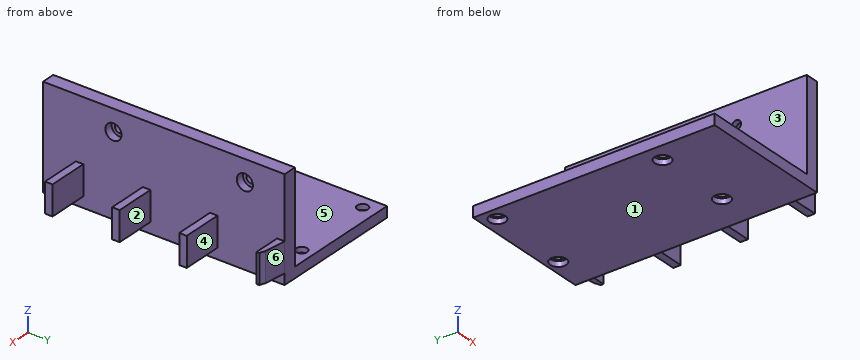
```python
from build123d import *

# Parameters (mm, degrees)
EXTRUDE_1_DEPTH     = 38
EXTRUDE_1_2_DEPTH   = 38
EXTRUDE_7_DEPTH     = 38
SKETCH_13_W         = 45
SKETCH_13_H         = 4
EXTRUDE_9_DEPTH     = 90
SKETCH_1_4_W        = 5
SKETCH_1_4_H        = 2.2
EXTRUDE_10_DEPTH    = 38
SKETCH_11_R         = 1.75
CUT_EXTRUDE_2_DEPTH = 38
CUT_EXTRUDE_START   = -2
SKETCH_11_3_R       = 3
SKETCH_11_3_R_2     = 1.75
CUT_EXTRUDE_3_DEPTH = 38
SKETCH_15_R         = 2
CUT_EXTRUDE_4_DEPTH = 38
SKETCH_15_3_R       = 3
SKETCH_15_3_R_2     = 2
CUT_EXTRUDE_5_DEPTH = 38
SKETCH_17_W         = 15
SKETCH_17_H         = 2.8
EXTRUDE_12_DEPTH    = 23
SKETCH_18_W         = 2
SKETCH_18_H         = 1
CUT_EXTRUDE_6_DEPTH = 40
SKETCH_17_2_W       = 15
SKETCH_17_2_H       = 2.8
SKETCH_17_2_W_2     = 10
SKETCH_17_2_H_2     = 3.8
CUT_EXTRUDE_7_DEPTH = 23
SKETCH_20_W         = 15
SKETCH_20_H         = 4
CUT_EXTRUDE_8_DEPTH = 89
SKETCH_17_4_W       = 5
SKETCH_17_4_H       = 10
EXTRUDE_13_DEPTH    = 38


with BuildPart() as part:
    # Sketch 1 → Extrude 1 (new body)
    with BuildSketch(Plane.XY):
        Polygon((15, -3.8), (15, -1.8), (13, -1), (13, -3.8), align=None)
    extrude(amount=EXTRUDE_1_DEPTH)



with BuildPart() as body_2:
    # Sketch 1 → Extrude 1 2 (new body)
    with BuildSketch(Plane.XY):
        Polygon((5, -75), (5, -52.8), (20, -52.8), (20, -50), (5, -50), (5, -27.8), (20, -27.8), (20, -25), (5, -25), (5, 0), (0, 0), (0, -77.8), (20, -77.8), (20, -75), align=None)
    extrude(amount=EXTRUDE_1_2_DEPTH)


with BuildPart() as part_1:
    add(part.part)

    add(body_2.part)  # Extrude 7 merges body 2
    # Sketch 1_3 → Extrude 7 (add)
    with BuildSketch(Plane.XY):
        Polygon((13, -2.8), (13, -1), (5, 0), (5, -0.74611229), (5, -2.8), align=None)
    extrude(amount=EXTRUDE_7_DEPTH)

    # Sketch 13 → Extrude 9 (add)
    with BuildSketch(Plane(origin=(0, 0, 0), x_dir=(1, 0, 0), z_dir=(0, 1, 0))):
        with Locations((-22.5, -2)):
            Rectangle(SKETCH_13_W, SKETCH_13_H)
    extrude(amount=-EXTRUDE_9_DEPTH)

    # Sketch 1_4 → Extrude 10 (add)
    with BuildSketch(Plane.XY):
        with Locations((2.5, -78.9)):
            Rectangle(SKETCH_1_4_W, SKETCH_1_4_H)
    extrude(amount=EXTRUDE_10_DEPTH)

    # Sketch 11 → Cut-Extrude 2 (cut)
    with BuildSketch(Plane.ZY):
        with Locations((30, -63.769774624)):
            Circle(SKETCH_11_R)
        with Locations((30, -14.819294268)):
            Circle(SKETCH_11_R)
    extrude(amount=-CUT_EXTRUDE_2_DEPTH, mode=Mode.SUBTRACT)

    # Sketch 11_3 → Cut-Extrude 3 (cut)
    with BuildSketch(Plane.ZY.offset(CUT_EXTRUDE_START)):
        with Locations((30, -63.769774624)):
            Circle(SKETCH_11_3_R)
        with Locations((30, -63.769774624)):
            Circle(SKETCH_11_3_R_2, mode=Mode.SUBTRACT)
        with Locations((30, -14.819294268)):
            Circle(SKETCH_11_3_R)
        with Locations((30, -14.819294268)):
            Circle(SKETCH_11_3_R_2, mode=Mode.SUBTRACT)
    extrude(amount=-CUT_EXTRUDE_3_DEPTH, mode=Mode.SUBTRACT)

    # Sketch 15 → Cut-Extrude 4 (cut)
    with BuildSketch(Plane.XY.offset(4)):
        with Locations((-40, -5.284222689)):
            Circle(SKETCH_15_R)
        with Locations((-9, -4.284222689)):
            Circle(SKETCH_15_R)
        with Locations((-9, -65.284222689)):
            Circle(SKETCH_15_R)
        with Locations((-38, -65.284222689)):
            Circle(SKETCH_15_R)
    extrude(amount=-CUT_EXTRUDE_4_DEPTH, mode=Mode.SUBTRACT)

    # Sketch 15_3 → Cut-Extrude 5 (cut)
    with BuildSketch(Plane.XY.offset(4).offset(CUT_EXTRUDE_START)):
        with Locations((-40, -5.284222689)):
            Circle(SKETCH_15_3_R)
        with Locations((-40, -5.284222689)):
            Circle(SKETCH_15_3_R_2, mode=Mode.SUBTRACT)
        with Locations((-38, -65.284222689)):
            Circle(SKETCH_15_3_R)
        with Locations((-38, -65.284222689)):
            Circle(SKETCH_15_3_R_2, mode=Mode.SUBTRACT)
        with Locations((-9, -65.284222689)):
            Circle(SKETCH_15_3_R)
        with Locations((-9, -65.284222689)):
            Circle(SKETCH_15_3_R_2, mode=Mode.SUBTRACT)
        with Locations((-9, -4.284222689)):
            Circle(SKETCH_15_3_R)
        with Locations((-9, -4.284222689)):
            Circle(SKETCH_15_3_R_2, mode=Mode.SUBTRACT)
    extrude(amount=-CUT_EXTRUDE_5_DEPTH, mode=Mode.SUBTRACT)

    # Sketch 17 → Extrude 12 (add)
    with BuildSketch(Plane.XY.offset(38)):
        with Locations((12.5, -26.4)):
            Rectangle(SKETCH_17_W, SKETCH_17_H)
        with Locations((12.5, -51.4)):
            Rectangle(SKETCH_17_W, SKETCH_17_H)
        with Locations((12.5, -76.4)):
            Rectangle(SKETCH_17_W, SKETCH_17_H)
    extrude(amount=-EXTRUDE_12_DEPTH)

    # Sketch 18 → Cut-Extrude 6 (cut)
    with BuildSketch(Plane.XY.offset(38)):
        with Locations((14, -3.3)):
            Rectangle(SKETCH_18_W, SKETCH_18_H)
    extrude(amount=-CUT_EXTRUDE_6_DEPTH, mode=Mode.SUBTRACT)

    # Sketch 17_2 → Cut-Extrude 7 (cut)
    with BuildSketch(Plane.XY.offset(38)):
        with Locations((12.5, -76.4)):
            Rectangle(SKETCH_17_2_W, SKETCH_17_2_H)
        with Locations((12.5, -51.4)):
            Rectangle(SKETCH_17_2_W, SKETCH_17_2_H)
        with Locations((12.5, -26.4)):
            Rectangle(SKETCH_17_2_W, SKETCH_17_2_H)
        with Locations((10, -1.9)):
            Rectangle(SKETCH_17_2_W_2, SKETCH_17_2_H_2)
    extrude(amount=-CUT_EXTRUDE_7_DEPTH, mode=Mode.SUBTRACT)

    # Sketch 20 → Cut-Extrude 8 (cut)
    with BuildSketch(Plane(origin=(0, 0, 0), x_dir=(1, 0, 0), z_dir=(0, 1, 0))):
        with Locations((12.5, -2)):
            Rectangle(SKETCH_20_W, SKETCH_20_H)
    extrude(amount=-CUT_EXTRUDE_8_DEPTH, mode=Mode.SUBTRACT)

    # Sketch 17_4 → Extrude 13 (add)
    with BuildSketch(Plane.XY.offset(38)):
        with Locations((2.5, -85)):
            Rectangle(SKETCH_17_4_W, SKETCH_17_4_H)
    extrude(amount=-EXTRUDE_13_DEPTH)


solid = part_1.part
```
Work out the finished part from the listing and answer in its coordinate system (mm). Face numbers are marked on the shaded views. A direction names the side the tool comes from. Round coordinates to 2 decimals unless told otherwise and drop trailing zeros. Loops run counter-clockwise (first coordinate to the right, second up) from the corner with the lowest first, then second, coordinate; pieces in that order, holes last. Notation, with made-up numbers: (5, 25.25) -> (32, 25.25) arc R20 ccw to (32, 51.25) -> close; hole circle Ø9 at (10.5, -22.75). An arc over 180 degrees is marked (long way). Write each question's results on one line, items separated by ' | '. Start each with the question number.
1. For a pull along Y with two mould halves and no side action, classify the marked faces 4, 5 and 6 as +Y half, -Y half, draft (parallel to the pull), parting line (faces both ways), or undercut.
2. A tool of negligible diameter and unlimited length cuts with its end or side. For the marked faces 1, 2 and 3, from which of +Z, -Z, +X, -X, +Y, -Y can it reach the whole face along a straight path? Write none if from no direction.
3. Given pin 1 Ø1 at (x, z) = (4.5, 28) entering from +Y; pin 2 Ø0.8 at (x, y) = (15, -51) entering from +Z; pin 3 Ø2.5 at (x, y) = (-38, -65.28) entering from -Z; pin 4 Ø5 at (y, z) = (-63.77, 30) entering from -X, each flat-ended and moving along its own axis, determine where each tip first touches the part or whether it passes through.
4. Section D-D (z = 6) is taken. Determine the outline of the cut face in (x, y).
5. Section A-A (z = 30) is taken. Determine the outline of the cut face in (x, y), plus the area to 3 significant figures.
6. Find the intervals of material crossed by probe 1 along Y at (x, z) = (-9, 3.1); probe 2 along Y at (x, z) = (1, 30); probe 3 along Y at (x, z) = (11.5, 5.5), in increasing order. Write a range as from..to.
7. Section C-C (y = -9.5) is taken. Determine the outline of the cut face in (x, z), plus the area to 3 significant figures.
8. Section B-B (x = -9) is taken. Determine the outline of the cut face in (y, z).
Evaluation:
1) face 4: undercut | face 5: draft | face 6: +Y half
2) face 1: -Z, +X, -X, +Y, -Y | face 2: +Z, -Z, +X | face 3: +Z, -X, +Y, -Y
3) pin 1: stops at y = 0 | pin 2: stops at z = 15 | pin 3: passes through | pin 4: stops at x = 0
4) outline: (0, -90) -> (5, -90) -> (5, -77.8) -> (20, -77.8) -> (20, -75) -> (5, -75) -> (5, -52.8) -> (20, -52.8) -> (20, -50) -> (5, -50) -> (5, -27.8) -> (20, -27.8) -> (20, -25) -> (5, -25) -> (5, -2.8) -> (15, -2.8) -> (15, -1.8) -> (13, -1) -> (5, 0) -> (0, 0) -> close
5) outline: (0, -90) -> (5, -90) -> (5, -66.77) -> (2, -66.77) -> (2, -65.52) -> (0, -65.52) -> close; (0, -62.02) -> (2, -62.02) -> (2, -60.77) -> (5, -60.77) -> (5, -17.82) -> (2, -17.82) -> (2, -16.57) -> (0, -16.57) -> close; (0, -13.07) -> (2, -13.07) -> (2, -11.82) -> (5, -11.82) -> (5, 0) -> (0, 0) -> close | area: 400 mm2
6) probe 1: y = -90..-67.28, -63.28..-6.28, -2.28..0 | probe 2: y = -90..-65.52, -62.02..-16.57, -13.07..0 | probe 3: y = -77.8..-75, -52.8..-50, -27.8..-25, -2.8..-0.81
7) outline: (-45, 0) -> (5, 0) -> (5, 38) -> (0, 38) -> (0, 4) -> (-45, 4) -> close | area: 370 mm2
8) outline: (-90, 0) -> (-68.28, 0) -> (-68.28, 2) -> (-67.28, 2) -> (-67.28, 4) -> (-90, 4) -> close; (-63.28, 2) -> (-62.28, 2) -> (-62.28, 0) -> (-7.28, 0) -> (-7.28, 2) -> (-6.28, 2) -> (-6.28, 4) -> (-63.28, 4) -> close; (-2.28, 2) -> (-1.28, 2) -> (-1.28, 0) -> (0, 0) -> (0, 4) -> (-2.28, 4) -> close
